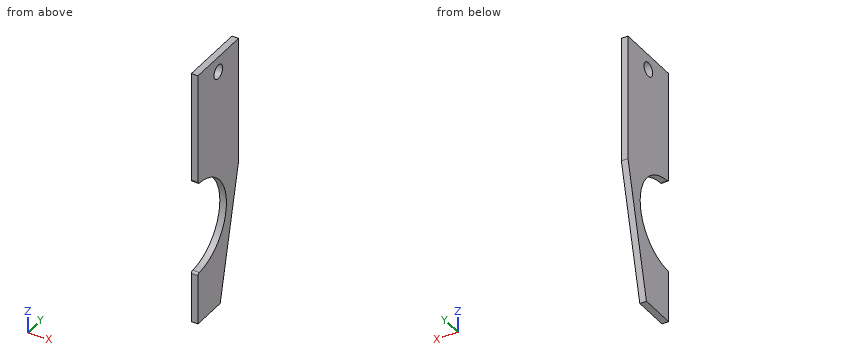
from build123d import *

# Parameters (mm, degrees)
BOSS_EXTRUDE1_DEPTH = 3
SKETCH2_R           = 3.175
CUT_EXTRUDE1_DEPTH  = 4
FILLET2_R           = 1


with BuildPart() as part:
    # Sketch1 → Boss-Extrude1 (new body)
    with BuildSketch(Plane(origin=(0, 0, 0), x_dir=(0, 0, -1), z_dir=(1, 0, 0))):
        with BuildLine():
            Line((0, 0), (57.50407585, 0))
            Line((57.50407585, 0), (116.474786715, -13.615081165))
            Line((116.474786715, -13.615081165), (116.474786715, -30))
            Line((116.474786715, -30), (92.883246032, -30))
            ThreePointArc((92.883246032, -30), (71.883246032, -9), (50.883246032, -30))
            Line((50.883246032, -30), (0, -30))
            Line((0, -30), (0, 0))
        make_face()
    extrude(amount=BOSS_EXTRUDE1_DEPTH)

    # Sketch2 → Cut-Extrude1 (cut, through all)
    with BuildSketch(Plane(origin=(3, 0, 0), x_dir=(0, 0, -1), z_dir=(1, 0, 0))):
        with Locations((6.900903962, -15)):
            Circle(SKETCH2_R)
    extrude(amount=-CUT_EXTRUDE1_DEPTH, mode=Mode.SUBTRACT)

    # Fillet2
    fillet2_edges = [part.edges().sort_by_distance(p)[0] for p in [
        (1.5, -30, -92.883246032),
        (1.5, -30, -50.883246032),
    ]]
    fillet(fillet2_edges, radius=FILLET2_R)


solid = part.part
Check sheet for the modelled part. Datum: model origin and axes. Units: mm. Round coordinates to 2 decimals unless told otherwise and drop trailing zeros. Loops run counter-clockwise (first coordinate to the right, second up) from the corner with the lowest first, then second, coordinate; pieces in that order, holes last. Notation, with made-up numbers: (4.25, -1.75) -> (25.25, -1.75) arc R30 cw to (25.25, 27.25) -> close; hole circle Ø4 at (-18.75, 35.25). An arc over 180 degrees is marked (long way). Put each result on its own line as item: value. Start each with the question number.
1. Section check A-A (y = -21.75). Enter the section's corners in (x, z), plus the area to 3 significant figures.
2. Scan lines: probe 1 along Z at (x, y) = (0.2, -27.5); probe 2 along Z at (x, y) = (0.4, -15.75); probe 3 along Y at (x, z) = (2.15, -50). Record each from-to range of solid material in increasing order.
3. Gauge pin test, flat end, axial feed: pin 1 (6 mm diameter, centred on y = -25.5, z = -24, fed in from -X). Record the tip position at first contact, or that the pin passes through.
4. Section check D-D (z = -74.5). Enter the section's corners in (x, y), plus the area to 3 significant figures.
5. Section check C-C (y = -15). Enter the section's corners in (x, z), plus the area to 3 significant figures.
Findings:
1. outline: (0, -116.47) -> (3, -116.47) -> (3, -91.19) -> (0, -91.19) -> close; (0, -52.57) -> (3, -52.57) -> (3, 0) -> (0, 0) -> close
1. area: 234 mm^2
2. probe 1: z = -116.47 to -92.73, -51.03 to 0
2. probe 2: z = -116.47 to -87.31, -56.46 to -9.99, -3.82 to 0
2. probe 3: y = -30 to 0
3. pin 1: stops at x = 0
4. outline: (0, -9.16) -> (3, -9.16) -> (3, -3.92) -> (0, -3.92) -> close
4. area: 15.7 mm^2
5. outline: (0, -116.47) -> (3, -116.47) -> (3, -86.58) -> (0, -86.58) -> close; (0, -57.19) -> (3, -57.19) -> (3, -10.08) -> (0, -10.08) -> close; (0, -3.73) -> (3, -3.73) -> (3, 0) -> (0, 0) -> close
5. area: 242 mm^2
